from build123d import *

# Parameters (mm, degrees)
F1_DEPTH = 75


# Not quite as in the source:
# - ends of sketch curves that miss each other by under 0.0002 mm in the source are joined


with BuildPart() as f1:
    # F0 (on Top) → F1 (new body, symmetric)
    with BuildSketch(Plane.XY):
        Polygon((7.5, 1.5), (7.5, 7.5), (1.5, 7.5), (1.5, 6), (3, 6), (3, 3.5), (1.1461396934, 2.7563427575), (1.1461396934, 2.42764467), (-1.1461396934, 2.42764467), (-1.1461396934, 2.7563427575), (-3, 3.5), (-3, 6), (-1.5, 6), (-1.5, 7.5), (-7.5, 7.5), (-7.5, 1.5), (-6, 1.5), (-6, 3), (-3.5, 3), (-2.7563427575, 1.1461396934), (-2.42764467, 1.1461396934), (-2.42764467, -1.1461396934), (-2.7563427575, -1.1461396934), (-3.5, -3), (-6, -3), (-6, -1.5), (-7.5, -1.5), (-7.5, -7.5), (-1.5, -7.5), (-1.5, -6), (-3, -6), (-3, -3.5), (-1.1461396934, -2.7563427575), (-1.1461396934, -2.42764467), (1.1461396934, -2.42764467), (1.1461396934, -2.7563427575), (3, -3.5), (3, -6), (1.5, -6), (1.5, -7.5), (7.5, -7.5), (7.5, -1.5), (6, -1.5), (6, -3), (3.5, -3), (2.7563427575, -1.1461396934), (2.42764467, -1.1461396934), (2.42764467, 1.1461396934), (2.7563427575, 1.1461396934), (3.5, 3), (6, 3), (6, 1.5), align=None)
    extrude(amount=F1_DEPTH, both=True)


solid = f1.part
The listing builds one solid part. Answer for the finished solid, in the listing's coordinates (mm). A direction names the side the tool comes from. Coordinates: 2 decimals unless noted, no trailing zeros. Write each loop counter-clockwise with the first axis right and the second up, starting at its lowest first coordinate (ties: lowest second). Pieces come first, ordered by that corner, then holes. Notation, with made-up numbers: (23.25, 89) - (78.25, 89) arc R26 cw to (78.25, 107) - close; hole circle Ø4 at (53, -38.75). An arc over 180 degrees is marked (long way). Answer as CSV lines item,"result".
1. Find section A-A (x = 4.75). Give the vertices of the cut face in (y, z).
Computed values:
outline,"(-7.5, -75) - (-3, -75) - (-3, 75) - (-7.5, 75) - close; (3, -75) - (7.5, -75) - (7.5, 75) - (3, 75) - close"
2. A tool of negligible diameter and unlimited length cuts with its end or side. For faces 1 (the flat face through (-5, 3, 1)), 2 (the flat face through (0, 2.428, 1)), 3 (the flat face through (2.428, 0, 1)), from which of +Z, -Z, +X, -X, +Y, -Y can it reach the whole face along a straight path? Write none if from no direction.
Computed values:
face 1,"+Z, -Z"
face 2,"+Z, -Z, +Y"
face 3,"+Z, -Z, +X"
3. Straight lines are drawn through the part: line 1 (Y direction, x = 6.75, z = 43); line 2 (X direction, y = -4.25, z = 42); line 3 (X direction, y = 1.75, z = -24). For each, find the intervals that lie inside material, in ascending order. Write a range as [from, to].
Computed values:
line 1,"y = [-7.5, -1.5], [1.5, 7.5]"
line 2,"x = [-7.5, -3], [3, 7.5]"
line 3,"x = [-7.5, -6], [-3, 3], [6, 7.5]"
4. Determine the mould class of faces 4 (the flat face through (5, 3, 1)), 5 (the flat face through (-2.428, 0, 1)), 6 (the flat face through (-4, 7.5, 1)) for opening direction X: +X half, -X half, draft (parallel to the pull), parting line (faces both ways), or undercut.
Computed values:
face 4,"undercut"
face 5,"-X half"
face 6,"draft"
5. Given P1, Ø1.5, axis at y = 1, z = -7, coming from the +X side; P2, Ø1.8, axis at x = -0.5, z = 27.5, coming from the -Y side; P3, Ø0.7, axis at y = 0, z = 30.5, coming from the +X side, each flat-ended and moving along its own axis, determine where each tip first touches the part or whether it passes through.
Computed values:
P1,"stops at x = 7.5"
P2,"stops at y = -2.86"
P3,"stops at x = 2.43"
